Work out the finished part from the listing and answer in its coordinate system (mm). Face numbers are marked on the shaded views. A direction names the side the tool comes from. Round coordinates to 2 decimals unless told otherwise and drop trailing zeros. Write each loop counter-clockwise with the first axis right and the second up, starting at its lowest first coordinate (ties: lowest second). Pieces come first, ordered by that corner, then holes.
1. Determine the mould class of the marked faces 3, 4 and 5 for opening direction X: pulls with the +X half, pulls with the -X half, needs draft (parallel to the pull), parting line crosses it, or undercut.
2. Find section B-B (x = 19). Write down the section's boundary in (y, z).
3. Flat-ended cylindrical pins translate along their axes: pin 1 Ø7.5 at (x, y) = (0, 0) entering from -Z; pin 2 Ø1.5 at (x, y) = (2.5, -1) entering from -Z; pin 3 Ø4 at (x, y) = (-0.5, -1.5) entering from -Z. Find the tip coordinate at first contact, or state that the pin passes through.
4. Find section A-A (x = 0). Write down the section's boundary in (y, z).
5. Straight lines are drawn through the part: probe 1 along X at (y, z) = (0, 4.55); probe 2 along Z at (x, y) = (5.5, 2); probe 3 along Z at (x, y) = (17.5, 0). For each, find the intervals that lie inside material, in ascending order.
6. A tool of negligible diameter and unlimited length cuts with its end or side. For the marked faces 1 and 2, from which of +Z, -Z, +X, -X, +Y, -Y can it reach the whole face along a straight path? Write none if from no direction.
Autodesk Inventor part; units mm, degrees
ref_plane "th1_XY" through (23.8252, 3.175, 0) normal (0, 0, 1) x (1, 0, 0)
ref_plane "th1_YZ" through (23.8252, 3.175, 0) normal (1, 0, 0) x (0, 1, 0)
ref_plane "th1_ZX" through (23.8252, 3.175, 0) normal (0, 1, 0) x (0, 0, 1)
sketch "Sketch_1" plane through (0, 0, 0) normal (0, 0, 1) x (1, 0, 0)
  line L0 (-6.35, 6.35) -> (-6.35, -6.35)
  line L1 (-6.35, -6.35) -> (23.8252, -6.35)
  line L2 (23.8252, -6.35) -> (23.8252, 6.35)
  line L3 (23.8252, 6.35) -> (-6.35, 6.35)
extrude "Extrusion1" add sketch "Sketch_1" along normal mid plane 12.7
sketch "Sketch_2" plane through (0, 0, 0) normal (0, 1, 0) x (-1, 0, 0)
  line L0 (6.35, -3.3338) -> (6.35, 3.3338)
  line L1 (6.35, 3.3338) -> (-11.1252, 3.3338)
  line L2 (-11.1252, 3.3338) -> (-11.1252, -3.3338)
  line L3 (-11.1252, -3.3338) -> (6.35, -3.3338)
extrude "Extrusion2" cut sketch "Sketch_2" along normal mid plane 12.7
sketch "Sketch_3" plane through (0, 0, 0) normal (0, 0, 1) x (1, 0, 0)
  line L0 (23.8252, 0) -> (12.6492, 0)
  line L1 (12.6492, 0) -> (12.6492, 2.6835)
  line L2 (12.6492, 2.6835) -> (23.3337, 2.6835)
  line L3 (23.3337, 2.6835) -> (23.8252, 3.175)
  line L4 (23.8252, 3.175) -> (23.8252, 0)
  line L5 (23.8252, 0) -> (12.6492, 0)
revolve "Revolution1" cut sketch "Sketch_3" angle 360 about axis through (23.8252, 0, 0) along (1, 0, 0)
thread "Thread1"
sketch "Sketch_4" plane through (0, 0, 0) normal (0, 0, 1) x (1, 0, 0)
  line L0 (12.6492, 0) -> (11.1252, 0)
  line L1 (11.1252, 0) -> (11.1252, 2.7051)
  line L2 (11.1252, 2.7051) -> (12.6492, 2.7051)
  line L3 (12.6492, 2.7051) -> (12.6492, 0)
  line L4 (12.6492, 0) -> (11.1252, 0)
revolve "Revolution2" cut sketch "Sketch_4" angle 360 about axis through (12.6492, 0, 0) along (1, 0, 0)
sketch "Sketch_5" plane through (0, 0, 0) normal (1, 0, 0) x (0, 1, 0)
  line L0 (0, -6.35) -> (0, 6.35)
  line L1 (0, 6.35) -> (4.337, 6.35)
  line L2 (4.337, 6.35) -> (3.194, 5.207)
  line L3 (3.194, 5.207) -> (3.194, -5.207)
  line L4 (3.194, -5.207) -> (4.337, -6.35)
  line L5 (4.337, -6.35) -> (0, -6.35)
  line L6 (0, -6.35) -> (0, 6.35)
revolve "Revolution3" cut sketch "Sketch_5" angle 360 about axis through (0, 0, -6.35) along (0, 0, -1)
sketch "Sketch_9" plane through (0, 0, 0) normal (0, 0, 1) x (1, 0, 0)
  line L0 (30.1752, 0) -> (23.8252, 0)
  line L1 (23.8252, 0) -> (23.8252, 6.35)
  arc A0 (23.8252, 6.35) -> (21.2852, 12.7) centre (6.6802, 3.175) ccw
  line L2 (21.2852, 12.7) -> (30.1752, 12.7)
  line L3 (30.1752, 12.7) -> (30.1752, 0)
  line L4 (30.1752, 0) -> (23.8252, 0)
revolve "Revolution4" cut sketch "Sketch_9" angle 360 about axis through (30.1752, 0, 0) along (1, 0, 0)
sketch "Sketch_10" plane through (0, 0, 0) normal (0, 0, 1) x (1, 0, 0)
  line L0 (-6.35, 0) -> (-12.7, 0)
  line L1 (-12.7, 0) -> (-12.7, 12.7)
  line L2 (-12.7, 12.7) -> (-3.81, 12.7)
  arc A0 (-3.81, 12.7) -> (-6.35, 6.35) centre (10.795, 3.175) ccw
  line L3 (-6.35, 6.35) -> (-6.35, 0)
  line L4 (-6.35, 0) -> (-12.7, 0)
revolve "Revolution5" cut sketch "Sketch_10" angle 360 about axis through (-6.35, 0, 0) along (1, 0, 0)
ref_plane "th1_XY" through (23.8252, 3.175, 0) normal (0, 0, 1) x (1, 0, 0)
ref_plane "th1_YZ" through (23.8252, 3.175, 0) normal (1, 0, 0) x (0, 1, 0)
ref_plane "th1_ZX" through (23.8252, 3.175, 0) normal (0, 1, 0) x (0, 0, 1)
ref_plane "th2_XY" through (23.8252, -3.175, 0) normal (0, 0, 1) x (1, 0, 0)
ref_plane "th2_YZ" through (23.8252, -3.175, 0) normal (1, 0, 0) x (0, 1, 0)
ref_plane "th2_ZX" through (23.8252, -3.175, 0) normal (0, 1, 0) x (0, 0, 1)
ref_plane "rod_clevis_body_XY" through (0, 0, 0) normal (0, 0, 1) x (1, 0, 0)
ref_plane "rod_clevis_body_YZ" through (0, 0, 0) normal (1, 0, 0) x (0, 1, 0)
ref_plane "rod_clevis_body_ZX" through (0, 0, 0) normal (0, 1, 0) x (0, 0, 1)
ref_plane "piston_rod_clevis_XY" through (23.8252, 0, 0) normal (1, 0, 0) x (0, 0, -1)
ref_plane "piston_rod_clevis_YZ" through (23.8252, 0, 0) normal (0, 0, -1) x (0, 1, 0)
ref_plane "piston_rod_clevis_ZX" through (23.8252, 0, 0) normal (0, 1, 0) x (1, 0, 0)
ref_plane "dummy_XY" through (0, 0, 0) normal (0, 0, 1) x (1, 0, 0)
ref_plane "dummy_YZ" through (0, 0, 0) normal (1, 0, 0) x (0, 1, 0)
ref_plane "dummy_ZX" through (0, 0, 0) normal (0, 1, 0) x (0, 0, 1)
ref_plane "l11_XY" through (23.8252, 6.35, 0) normal (0, 0, 1) x (1, 0, 0)
ref_plane "l11_YZ" through (23.8252, 6.35, 0) normal (1, 0, 0) x (0, 1, 0)
ref_plane "l11_ZX" through (23.8252, 6.35, 0) normal (0, 1, 0) x (0, 0, 1)
ref_plane "l12_XY" through (0, 6.35, 0) normal (0, 0, 1) x (1, 0, 0)
ref_plane "l12_YZ" through (0, 6.35, 0) normal (1, 0, 0) x (0, 1, 0)
ref_plane "l12_ZX" through (0, 6.35, 0) normal (0, 1, 0) x (0, 0, 1)
ref_plane "l1_XY" through (23.8252, 6.35, 0) normal (0, 0, 1) x (1, 0, 0)
ref_plane "l1_YZ" through (23.8252, 6.35, 0) normal (1, 0, 0) x (0, 1, 0)
ref_plane "l1_ZX" through (23.8252, 6.35, 0) normal (0, 1, 0) x (0, 0, 1)
ref_plane "h1_XY" through (-6.35, 6.35, 0) normal (0, 0, 1) x (1, 0, 0)
ref_plane "h1_YZ" through (-6.35, 6.35, 0) normal (1, 0, 0) x (0, 1, 0)
ref_plane "h1_ZX" through (-6.35, 6.35, 0) normal (0, 1, 0) x (0, 0, 1)
ref_plane "l2_XY" through (-6.35, 6.35, 0) normal (0, 0, 1) x (1, 0, 0)
ref_plane "l2_YZ" through (-6.35, 6.35, 0) normal (1, 0, 0) x (0, 1, 0)
ref_plane "l2_ZX" through (-6.35, 6.35, 0) normal (0, 1, 0) x (0, 0, 1)
ref_plane "h2_XY" through (-6.35, -6.35, 0) normal (0, 0, 1) x (1, 0, 0)
ref_plane "h2_YZ" through (-6.35, -6.35, 0) normal (1, 0, 0) x (0, 1, 0)
ref_plane "h2_ZX" through (-6.35, -6.35, 0) normal (0, 1, 0) x (0, 0, 1)
ref_plane "w11_XY" through (-6.35, 0, -3.3338) normal (0, 1, 0) x (1, 0, 0)
ref_plane "w11_YZ" through (-6.35, 0, -3.3338) normal (1, 0, 0) x (0, 0, -1)
ref_plane "w11_ZX" through (-6.35, 0, -3.3338) normal (0, 0, -1) x (0, 1, 0)
ref_plane "w12_XY" through (-6.35, 0, 3.3338) normal (0, 1, 0) x (1, 0, 0)
ref_plane "w12_YZ" through (-6.35, 0, 3.3338) normal (1, 0, 0) x (0, 0, -1)
ref_plane "w12_ZX" through (-6.35, 0, 3.3338) normal (0, 0, -1) x (0, 1, 0)
ref_plane "l21_XY" through (23.8252, 0, 0) normal (0, 1, 0) x (1, 0, 0)
ref_plane "l21_YZ" through (23.8252, 0, 0) normal (1, 0, 0) x (0, 0, -1)
ref_plane "l21_ZX" through (23.8252, 0, 0) normal (0, 0, -1) x (0, 1, 0)
ref_plane "l22_XY" through (11.1252, 0, 0) normal (0, 1, 0) x (1, 0, 0)
ref_plane "l22_YZ" through (11.1252, 0, 0) normal (1, 0, 0) x (0, 0, -1)
ref_plane "l22_ZX" through (11.1252, 0, 0) normal (0, 0, -1) x (0, 1, 0)
ref_plane "w1_XY" through (23.8252, 0, -6.35) normal (0, 1, 0) x (1, 0, 0)
ref_plane "w1_YZ" through (23.8252, 0, -6.35) normal (1, 0, 0) x (0, 0, -1)
ref_plane "w1_ZX" through (23.8252, 0, -6.35) normal (0, 0, -1) x (0, 1, 0)
ref_plane "w2_XY" through (23.8252, 0, 6.35) normal (0, 1, 0) x (1, 0, 0)
ref_plane "w2_YZ" through (23.8252, 0, 6.35) normal (1, 0, 0) x (0, 0, -1)
ref_plane "w2_ZX" through (23.8252, 0, 6.35) normal (0, 0, -1) x (0, 1, 0)
ref_plane "to_cylinder_XY" through (11.1252, 0, 0) normal (1, 0, 0) x (0, 0, -1)
ref_plane "to_cylinder_YZ" through (11.1252, 0, 0) normal (0, 0, -1) x (0, 1, 0)
ref_plane "to_cylinder_ZX" through (11.1252, 0, 0) normal (0, 1, 0) x (1, 0, 0)
properties part number "D-14055"
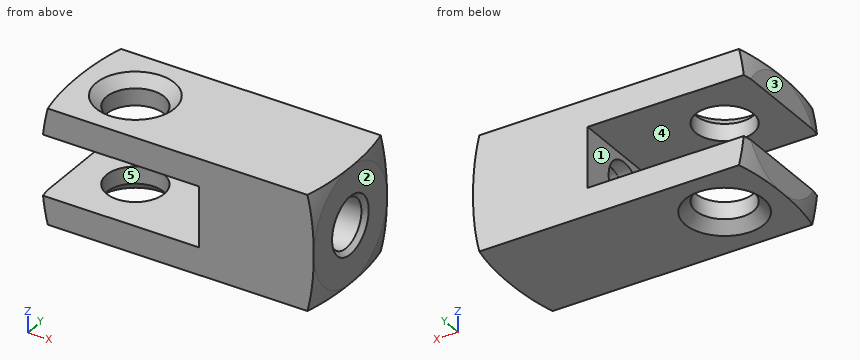
Worked answers:
1. face 3: pulls with the -X half
1. face 4: needs draft
1. face 5: undercut
2. outline: (-6.35, -6.35) - (6.35, -6.35) - (6.35, 6.35) - (-6.35, 6.35) - close; hole circle Ø5.37 at (0, 0)
3. pin 1: stops at z = -5.76
3. pin 2: stops at z = -5.46
3. pin 3: stops at z = -5.59
4. outline: (-6.35, -6.35) - (-4.34, -6.35) - (-3.19, -5.21) - (-3.19, -3.33) - (-6.35, -3.33) - close; (-6.35, 3.33) - (-3.19, 3.33) - (-3.19, 5.21) - (-4.34, 6.35) - (-6.35, 6.35) - close; (3.19, -5.21) - (4.34, -6.35) - (6.35, -6.35) - (6.35, -3.33) - (3.19, -3.33) - close; (3.19, 3.33) - (6.35, 3.33) - (6.35, 6.35) - (4.34, 6.35) - (3.19, 5.21) - close
5. probe 1: x = -6.35 to -3.19, 3.19 to 23.83
5. probe 2: z = -6.35 to -3.33, 3.33 to 6.35
5. probe 3: z = -6.35 to -2.68, 2.68 to 6.35
6. face 1: -X, +Y, -Y
6. face 2: +Z, -Z, +X, +Y, -Y
